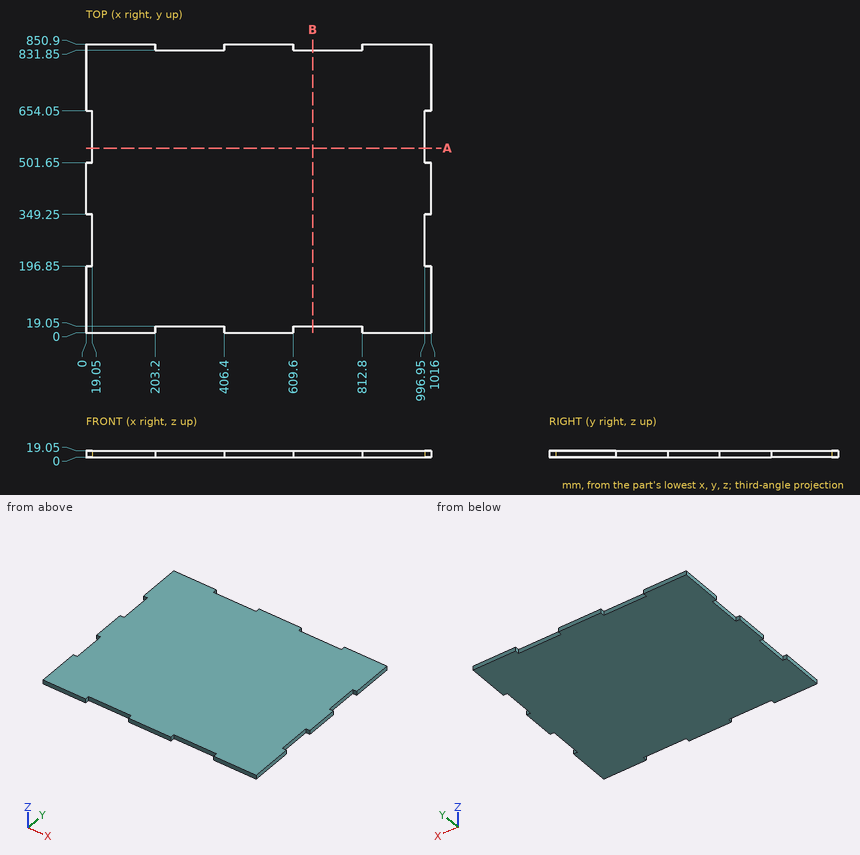
Could you check a few things on this drawing? It's one solid part, dimensions in mm from its lowest x, y, z. Give positions to 0.01 mm unless a question says otherwise; leave off trailing zeros. Order: outer loops, then holes, each group sorted by start corner. A loop starts at its lowest first (then second) coordinate and runs counter-clockwise, first axis right, second up. Notation, with made-up numbers: M 3,14 L 53,14 A18 ccw 53,35 Z; hole C -3,-27.5 d1. An arc over 180 degrees is marked long. Use one line per item in the form item = value. Start each with the question number.
Item 1: If we section it at B-B (x = 667): Write out the boundary of the cut face in (y, z).
Item 2: If we section it at A-A (y = 544): Write out the boundary of the cut face in (x, z), then the cut area to 3 significant figures.
Item 3: Will these pins go through, and if not, where does the flat tip stop? pin 1 Ø1 at (y, z) = (535.5, 2) entering from -X; pin 2 Ø9.5 at (y, z) = (569.5, 6) entering from +X; pin 3 Ø8 at (x, z) = (678, 5.5) entering from +Y.
Item 4: If I drill on line 1 along X through (y, z) = (282, 3.5); line 2 along Y through (x, z) = (765.5, 11), over which ranges is the centre line in solid material (lowest first)?
Outcome:
q1.outline = M 19.05,0 L 831.85,0 L 831.85,19.05 L 19.05,19.05 Z
q2.outline = M 19.05,0 L 996.95,0 L 996.95,19.05 L 19.05,19.05 Z
q2.area = 18,600 mm2
q3.pin_1 = 19.05
q3.pin_2 = 996.95
q3.pin_3 = 831.85
q4.line_1 = 19.05 to 996.95
q4.line_2 = 19.05 to 831.85
